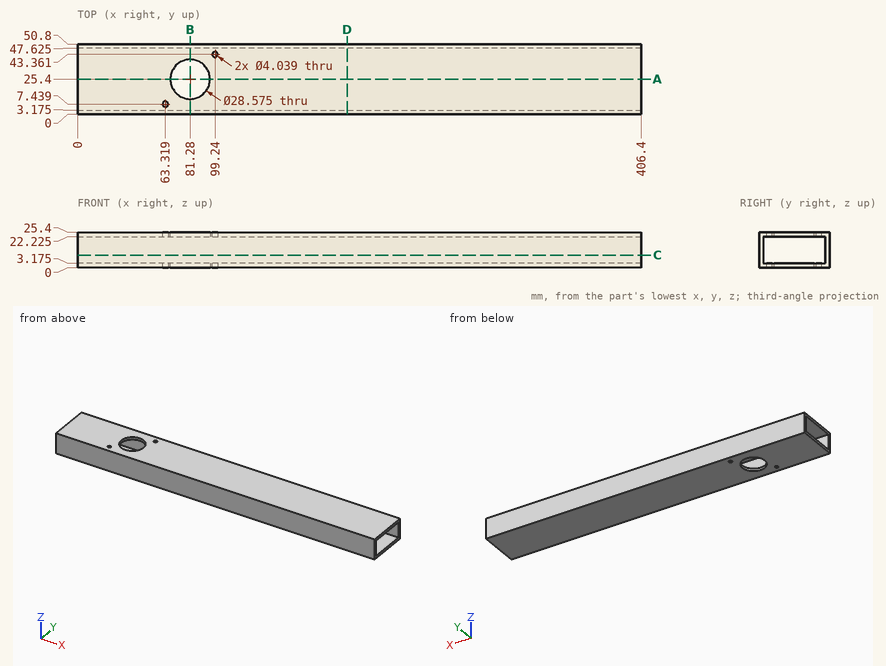
Job drawing, mm, ordinate dimensions from the low corner. One solid piece. Coordinates: 2 decimals unless noted, no trailing zeros. Order: outer loops, then holes, each group sorted by start corner. A loop starts at its lowest first (then second) coordinate and runs counter-clockwise, first axis right, second up. Notation, with made-up numbers: (-21.5, -8.5) - (3.5, -8.5) arc R8 cw to (3.5, 2.5) - close; hole circle Ø9 at (-31, -11.5). An arc over 180 degrees is marked (long way). Write each question's results on one line, items separated by ' | '. Start each with the question number.
Item 1: Band-saw the part on D-D on x = 194.5. Write the cut outline in (y, z) (1 decimal).
Item 2: Band-saw the part on A-A on y = 25.4. Write the cut outline in (x, z) (1 decimal), and give its area (3 significant figures).
Item 3: Wall check: probe 1 along Z at (x, y) = (243, 6.5) (1 decimal); probe 2 along Y at (x, z) = (72.5, 5.25) (1 decimal); probe 3 along Y at (x, z) = (81.28, 23.15). Give the ranges that are in metal, low to high. Write a range as [from, to].
Item 4: Flat gauge pin, fed straight in: pin 1 (17 mm diameter, centred on x = 81.28, y = 25.4, fed in from +Z). Where does the tip first touch, or does it go through?
Item 5: Band-saw the part on B-B on x = 81.28. Write the cut outline in (y, z) (1 decimal), and give its area (3 significant figures).
Item 6: Band-saw the part on C-C on z = 9. Write the cut outline in (x, y) (1 decimal), and give its area (3 significant figures).
Numbers:
1) outline: (0, 0) - (50.8, 0) - (50.8, 25.4) - (0, 25.4) - close; hole (3.2, 3.2) - (47.6, 3.2) - (47.6, 22.2) - (3.2, 22.2) - close
2) outline: (0, 0) - (67, 0) - (67, 3.2) - (0, 3.2) - close; (0, 22.2) - (67, 22.2) - (67, 25.4) - (0, 25.4) - close; (95.6, 0) - (406.4, 0) - (406.4, 3.2) - (95.6, 3.2) - close; (95.6, 22.2) - (406.4, 22.2) - (406.4, 25.4) - (95.6, 25.4) - close | area: 2,400 mm^2
3) probe 1: [0, 3.2], [22.2, 25.4] | probe 2: [0, 3.2], [47.6, 50.8] | probe 3: [0, 11.11], [39.69, 50.8]
4) pin 1: through
5) outline: (0, 0) - (11.1, 0) - (11.1, 3.2) - (3.2, 3.2) - (3.2, 22.2) - (11.1, 22.2) - (11.1, 25.4) - (0, 25.4) - close; (39.7, 0) - (50.8, 0) - (50.8, 25.4) - (39.7, 25.4) - (39.7, 22.2) - (47.6, 22.2) - (47.6, 3.2) - (39.7, 3.2) - close | area: 262 mm^2
6) outline: (0, 0) - (406.4, 0) - (406.4, 3.2) - (0, 3.2) - close; (0, 47.6) - (406.4, 47.6) - (406.4, 50.8) - (0, 50.8) - close | area: 2,580 mm^2
